Autodesk Inventor part; units mm, degrees
ref_plane "YZ Plane" through (0, 0, 0) normal (1, 0, 0) x (0, 1, 0)
ref_plane "XZ Plane" through (0, 0, 0) normal (0, 1, 0) x (-1, 0, 0)
ref_plane "XY Plane" through (0, 0, 0) normal (0, 0, 1) x (1, 0, 0)
sketch "Sketch1" plane through (0, 0, 0) normal (0, 0, 1) x (1, 0, 0)
  line L0 (39.835, -215.3282) -> (-188.765, -215.3282)
  line L1 (-188.765, -215.3282) -> (-188.765, -22.2882)
  line L2 (-188.765, -22.2882) -> (39.835, -22.2882)
  line L3 (39.835, -22.2882) -> (39.835, -215.3282)
  point P0 (0, 0)
  dimension "d0" = 228.6
  dimension "d1" = 193.04
extrude "Extrusion1" add sketch "Sketch1" along normal blind 3.175
sketch "Sketch2" plane through (0, 0, 3.175) normal (0, 0, 1) x (1, 0, 0)
  line L0 (-188.765, -215.3282) -> (39.835, -215.3282)
  line L1 (39.835, -215.3282) -> (39.835, -212.1532)
  line L2 (39.835, -212.1532) -> (-188.765, -212.1532)
  line L3 (-188.765, -212.1532) -> (-188.765, -215.3282)
  point P0 (0, 0)
  dimension "d4" = 228.6
  dimension "d5" = 3.175
extrude "Extrusion2" add sketch "Sketch2" along normal blind 63.5
fillet "Fillet1" radius 3.175 2 edges at (-74.465, -212.1532, 3.175) (-74.465, -215.3282, 0)
sketch "Sketch3" plane through (-188.765, -212.1532, 66.675) normal (0, 1, 0) x (1, 0, 0)
  line L0 (0, 60.325) -> (228.6, 60.325)
  line L1 (0, 60.325) -> (0, 0)
  line L2 (0, 0) -> (228.6, 0)
  line L3 (228.6, 60.325) -> (228.6, 0)
  circle A0 centre (12.7, 47.625) radius 3.175
  circle A1 centre (114.3, 30.1625) radius 3.175
  circle A2 centre (215.9, 47.625) radius 3.175
  circle A3 centre (57.15, 12.7) radius 3.175
  circle A4 centre (171.45, 12.7) radius 3.175
  point P0 (188.765, 66.675)
  dimension "d9" = 6.35
  dimension "d10" = 6.35
  dimension "d11" = 6.35
  dimension "d12" = 6.35
  dimension "d13" = 6.35
  dimension "d14" = 12.7
  dimension "d15" = 12.7
  dimension "d16" = 12.7
  dimension "d17" = 12.7
  dimension "d18" = 114.3
  dimension "d19" = 228.6
  dimension "d20" = 57.15
  dimension "d21" = 12.7
  dimension "d22" = 12.7
  dimension "d23" = 57.15
  dimension "d24" = 30.1625
  dimension "d25" = 60.325
extrude "Extrusion3" cut sketch "Sketch3" against normal blind 63.5 contours A0 | A1 | A2 | A3 | A4
sketch "Sketch4" plane through (0, 0, 3.175) normal (0, 0, 1) x (1, 0, 0)
  line L0 (39.835, -22.2882) -> (39.835, -208.9782)
  line L1 (-188.765, -22.2882) -> (39.835, -22.2882)
  line L2 (-188.765, -208.9782) -> (-188.765, -22.2882)
  circle A0 centre (-176.065, -34.9882) radius 3.175
  circle A1 centre (27.135, -34.9882) radius 3.175
  circle A2 centre (-176.065, -161.9882) radius 3.175
  circle A3 centre (27.135, -161.9882) radius 3.175
  point P0 (0, 0)
  dimension "d28" = 6.35
  dimension "d29" = 6.35
  dimension "d30" = 12.7
  dimension "d31" = 12.7
  dimension "d32" = 12.7
  dimension "d33" = 12.7
  dimension "d34" = 6.35
  dimension "d35" = 6.35
  dimension "d36" = 12.7
  dimension "d37" = 12.7
  dimension "d38" = 127
  dimension "d39" = 127
extrude "Extrusion4" cut sketch "Sketch4" against normal blind 63.5
equation "\"d18\" = 0.5 * d19"
equation "\"d20\" = 0.25 * d19"
equation "\"d22\" = d21"
equation "\"d23\" = d20"
equation "\"d24\" = 0.5 * d25"
equation "\"d37\" = d36"
equation "\"d39\" = d38"
properties part number "PowerDistributionStandmount"
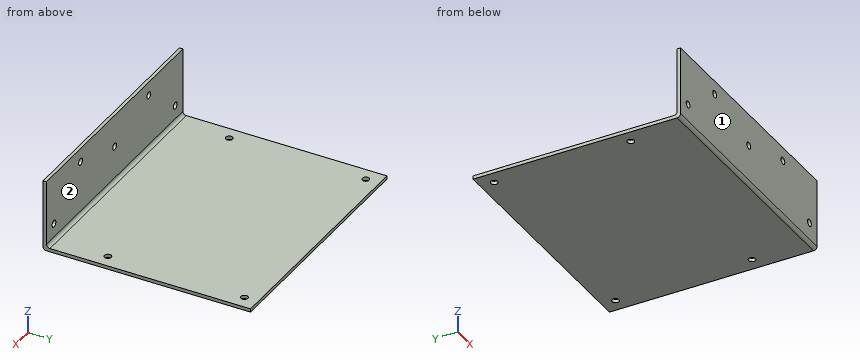
Part model, mm, in its own coordinate system. Face numbers are marked on the shaded views. A direction names the side the tool comes from. Coordinates: 2 decimals unless noted, no trailing zeros. Order: outer loops, then holes, each group sorted by start corner. A loop starts at its lowest first (then second) coordinate and runs counter-clockwise, first axis right, second up. Notation, with made-up numbers: M -16.5,-22 L 34.5,-22 A17 ccw 34.5,8 Z; hole C -16.5,-28.75 d9. An arc over 180 degrees is marked long. One line per question, with ' | ' between items.
Q1. Slice it at B-B (x = -60). Give the cut face in (y, z) (3 decimals), and give its area (3 significant figures).
A:
outline: M -215.328,3.175 A3.175 ccw -212.153,0 L -22.288,0 L -22.288,3.175 L -208.978,3.175 A3.175 cw -212.153,6.35 L -212.153,66.675 L -215.328,66.675 Z | area: 815 mm^2
Q2. 3-axis set-ups, long thin cutter, end or side, ignore diameter. For the marked faces 1 and 2: which of +Z, -Z, +X, -X, +Y, -Y reach the whole face in a straight line?
A:
face 1: +Z, -Z, +X, -X, -Y | face 2: +Z, +X, -X, +Y
Q3. Slice it at C-C (y = -50). Give the cut face in (x, z) (3 decimals), and give its area (3 significant figures).
A:
outline: M -188.765,0 L 39.835,0 L 39.835,3.175 L -188.765,3.175 Z | area: 726 mm^2
Q4. Drill centre lines: line 1 (X direction, y = -214.3, z = 19.05) (3 decimals); line 2 (Y direction, x = -46, z = 47.5); line 3 (Z direction, x = -1.5, y = -55.5) (3 decimals). Where is each one in solid material? Low to high.
A:
line 1: x = -188.765 to -179.24, -172.89 to 23.96, 30.31 to 39.835 | line 2: y = -215.33 to -212.15 | line 3: z = 0 to 3.175
Q5. Slice it at A-A (z = 19.05). Give the cut face in (x, y) (3 decimals), and give its area (3 significant figures).
A:
outline: M -188.765,-215.328 L -179.24,-215.328 L -179.24,-212.153 L -188.765,-212.153 Z; M -172.89,-215.328 L 23.96,-215.328 L 23.96,-212.153 L -172.89,-212.153 Z; M 30.31,-215.328 L 39.835,-215.328 L 39.835,-212.153 L 30.31,-212.153 Z | area: 685 mm^2
Q6. Pin check, flat tips, straight feed: P1, Ø18, axis at x = -36, z = 28, coming from the +Y side; P2, Ø7.5, axis at x = -176.06, y = -34.99, coming from the +Z side (3 decimals). Stop position of each tip, or through.
A:
P1: stops at y = -212.15 | P2: stops at z = 3.175
